Design review of the part built by this model. Coordinates are the model's own, in mm. A direction names the side the tool comes from. Round coordinates to 2 decimals unless told otherwise and drop trailing zeros. Loops run counter-clockwise (first coordinate to the right, second up) from the corner with the lowest first, then second, coordinate; pieces in that order, holes last. Notation, with made-up numbers: M 63.25,78.25 L 82.25,78.25 A31 ccw 82.25,115.25 Z; hole C -25.5,65.25 d5. An arc over 180 degrees is marked long. One line per item, written item: value. Start each with the question number.
Item 1: For faces 1 (the flat face through (68, -13.545, 8)), 2 (the flat face through (60.993, 27.798, 7.88)), 3 (the flat face through (50.546, 30, 6)), 4 (the cylindrical face through (21.97, -7.67, 1.93)), 5 (the cylindrical face through (48.735, -20.96, 1.878)), list the 3-axis set-ups (+Z, -Z, +X, -X, +Y, -Y) from which the entire face can be reached by the end or side of a thin tool; tool diameter is ignored.
Item 2: Clearance check with flat-ended pins moving along their axes: pin 1 (1.2 mm diameter, centred on x = -16.002, y = 19.05, fed in from +Z); pin 2 (3 mm diameter, centred on x = 49.5, z = 2, fed in from -Y); pin 3 (4 mm diameter, centred on x = 52, z = 1, fed in from +Y); pin 4 (8 mm diameter, centred on x = 15.24, y = -11.43, fed in from +Z). State where each tip first meets the part, or that it passes through.
Item 3: We need section B-B (z = 10.25). State how many separate pieces and enclosed holes the cut face has, then the cut area to 3 significant figures.
Item 4: We need section C-C (x = 42.5). Write out the cut boundary in (y, z) (3 decimals).
Item 5: For line 1 along Y through (x, z) = (0, 3); line 2 along Y through (x, z) = (-11, 1.75); line 3 along Y through (x, z) = (51, 7.5), list the stretches that pass through material, from the lowest coordinate up.
Item 6: We need section D-D (x = 15.24). Write out the cut boundary in (y, z) (3 decimals), then the cut area to 3 significant figures.
Item 7: We need section A-A (x = -41). Write out the cut boundary in (y, z) (3 decimals).
Item 8: Mouldability with a two-part tool opening along Y and no side actions: class faces 6 (the cylindrical face through (64.222, -32.664, 6.388)), 7 (the flat face through (1, 1, 0)), 8 (the cylindrical face through (6.5, -20.9, 1.9)) as released by +Y, released by -Y, zero draft, split by the parting line, or undercut.
from build123d import *

# Parameters (mm, degrees)
BOSS_EXTRUDE1_DEPTH     = 3.81
BOSS_EXTRUDE2_DEPTH     = 8.255
SKETCH3_W               = 64.77
SKETCH3_H               = 7.1
CUT_EXTRUDE1_DEPTH      = 0.635
CUT_EXTRUDE4_DEPTH      = 4.81
CUT_EXTRUDE5_DEPTH      = 4.81
SKETCH12_R              = 2.4257
CUT_EXTRUDE6_DEPTH      = 4.81
SKETCH4_R               = 1.143
CUT_EXTRUDE2_DEPTH      = 11.43
SKETCH17_R              = 2.413
CUT_EXTRUDE9_DEPTH      = 4.81
BOSS_EXTRUDE5_DEPTH     = 8.255
SKETCH20_W              = 69.85
SKETCH20_H              = 3.175
BOSS_EXTRUDE6_DEPTH     = 2.54
SKETCH21_R              = 1.02235
CUT_EXTRUDE10_DEPTH     = 13.065
SKETCH24_R              = 1.6383
CUT_EXTRUDE11_DEPTH     = 8.128
CIRPATTERN1_COUNT       = 2
CIRPATTERN1_ANGLE       = 15
MIRROR2_COPY_1_SKETCH_R = 1.6383
MIRROR2_COPY_1_DEPTH    = 8.128


with BuildPart() as part:
    # Sketch1 → Boss-Extrude1 (new body)
    with BuildSketch(Plane.XY):
        with BuildLine():
            Line((10.977415053, 19.05), (44.196, 19.05))
            ThreePointArc((44.196, 19.05), (48.686128061, 20.909871939), (50.546, 25.4))
            Line((50.546, 25.4), (50.546, 44.45))
            Line((50.546, 44.45), (61.579155694, 44.45))
            ThreePointArc((61.579155694, 44.45), (75.946, 0), (61.579155694, -44.45))
            Line((61.579155694, -44.45), (50.546, -44.45))
            Line((50.546, -44.45), (50.546, -25.4))
            ThreePointArc((50.546, -25.4), (48.686128061, -20.909871939), (44.196, -19.05))
            Line((44.196, -19.05), (10.977415053, -19.05))
            ThreePointArc((10.977415053, -19.05), (6.487286992, -20.909871939), (4.627415053, -25.4))
            Line((4.627415053, -25.4), (-71.572584947, -25.4))
            ThreePointArc((-71.572584947, -25.4), (-75.946, 0), (-71.572584947, 25.4))
            Line((-71.572584947, 25.4), (4.627415053, 25.4))
            ThreePointArc((4.627415053, 25.4), (6.487286992, 20.909871939), (10.977415053, 19.05))
        make_face()
    extrude(amount=BOSS_EXTRUDE1_DEPTH)

    # Sketch2 → Boss-Extrude2 (add)
    with BuildSketch(Plane.XY.offset(3.81)):
        with BuildLine():
            Line((61.865268471, 17.78), (60.095110466, 38.1))
            ThreePointArc((60.095110466, 38.1), (59.464196764, 40.158289632), (58.047089349, 41.778911391))
            Line((58.047089349, 41.778911391), (57.900800643, 44.704))
            Line((57.900800643, 44.704), (61.395010384, 44.704))
            ThreePointArc((61.395010384, 44.704), (69.822038137, 29.877715884), (74.728381149, 13.544887112))
            Line((74.728381149, 13.544887112), (60.759450402, 13.544887112))
            Line((60.759450402, 13.544887112), (60.759450402, 15.094127876))
            ThreePointArc((60.759450402, 15.094127876), (61.639191639, 16.302501703), (61.865268471, 17.78))
        make_face()
        with BuildLine():
            Line((58.651639318, 17.500047669), (56.881481313, 37.820047669))
            Line((56.881481313, 37.820047669), (50.546, 37.820047669))
            Line((50.546, 37.820047669), (50.546, 16.566735288))
            Line((50.546, 16.566735288), (57.366094516, 16.566735288))
            ThreePointArc((57.366094516, 16.566735288), (58.160401987, 16.824667019), (58.651639318, 17.500047669))
        make_face()
        with BuildLine():
            Line((60.759450402, -13.544887112), (74.728381149, -13.544887112))
            ThreePointArc((74.728381149, -13.544887112), (69.822038137, -29.877715884), (61.395010384, -44.704))
            Line((61.395010384, -44.704), (57.900800643, -44.704))
            Line((57.900800643, -44.704), (58.047089349, -41.778911391))
            ThreePointArc((58.047089349, -41.778911391), (59.464196764, -40.158289632), (60.095110466, -38.1))
            Line((60.095110466, -38.1), (61.865268471, -17.78))
            ThreePointArc((61.865268471, -17.78), (61.639191639, -16.302501703), (60.759450402, -15.094127876))
            Line((60.759450402, -15.094127876), (60.759450402, -13.544887112))
        make_face()
        with BuildLine():
            Line((50.546, -16.566735288), (57.366094516, -16.566735288))
            ThreePointArc((57.366094516, -16.566735288), (58.160401987, -16.824667019), (58.651639318, -17.500047669))
            Line((58.651639318, -17.500047669), (56.881481313, -37.820047669))
            Line((56.881481313, -37.820047669), (50.546, -37.820047669))
            Line((50.546, -37.820047669), (50.546, -16.566735288))
        make_face()
    extrude(amount=BOSS_EXTRUDE2_DEPTH)

    # Sketch3 → Cut-Extrude1 (cut)
    with BuildSketch(Plane.XY.offset(3.81)):
        with Locations((44.577, 0)):
            Rectangle(SKETCH3_W, SKETCH3_H)
    extrude(amount=-CUT_EXTRUDE1_DEPTH, mode=Mode.SUBTRACT)

    # Sketch9 → Cut-Extrude4 (cut, through all)
    with BuildSketch(Plane.XY.offset(3.81)):
        with BuildLine():
            Line((69.85, 11.17), (25.4, 11.17))
            ThreePointArc((25.4, 11.17), (21.971, 7.741), (25.4, 4.312))
            Line((25.4, 4.312), (69.85, 4.312))
            ThreePointArc((69.85, 4.312), (73.279, 7.741), (69.85, 11.17))
        make_face()
        with BuildLine():
            Line((69.85, -4.312), (25.4, -4.312))
            ThreePointArc((25.4, -4.312), (21.971, -7.741), (25.4, -11.17))
            Line((25.4, -11.17), (69.85, -11.17))
            ThreePointArc((69.85, -11.17), (73.279, -7.741), (69.85, -4.312))
        make_face()
    extrude(amount=-CUT_EXTRUDE4_DEPTH, mode=Mode.SUBTRACT)

    # Sketch10 → Cut-Extrude5 (cut, through all)
    with BuildSketch(Plane.XY.offset(3.81)):
        with BuildLine():
            Line((-10.922, 11.43), (-59.182, 11.43))
            ThreePointArc((-59.182, 11.43), (-61.42706403, 10.50006403), (-62.357, 8.255))
            Line((-62.357, 8.255), (-62.357, -8.255))
            ThreePointArc((-62.357, -8.255), (-61.42706403, -10.50006403), (-59.182, -11.43))
            Line((-59.182, -11.43), (-10.922, -11.43))
            ThreePointArc((-10.922, -11.43), (-8.67693597, -10.50006403), (-7.747, -8.255))
            Line((-7.747, -8.255), (-7.747, 8.255))
            ThreePointArc((-7.747, 8.255), (-8.67693597, 10.50006403), (-10.922, 11.43))
        make_face()
    extrude(amount=-CUT_EXTRUDE5_DEPTH, mode=Mode.SUBTRACT)

    # Sketch12 → Cut-Extrude6 (cut, through all)
    with BuildSketch(Plane.XY.offset(3.81)):
        with Locations((15.24, 11.43)):
            Circle(SKETCH12_R)
        with Locations((15.24, -11.43)):
            Circle(SKETCH12_R)
    extrude(amount=-CUT_EXTRUDE6_DEPTH, mode=Mode.SUBTRACT)

    # Sketch4 → Cut-Extrude2 (cut)
    with BuildSketch(Plane.XY.offset(3.175)):
        with Locations((19.812, 0)):
            Circle(SKETCH4_R)
        with Locations((34.798, 0)):
            Circle(SKETCH4_R)
        with Locations((49.784, 0)):
            Circle(SKETCH4_R)
        with Locations((64.77, 0)):
            Circle(SKETCH4_R)
    extrude(amount=-CUT_EXTRUDE2_DEPTH, mode=Mode.SUBTRACT)

    # Sketch17 → Cut-Extrude9 (cut, through all)
    with BuildSketch(Plane.XY.offset(3.81)):
        with Locations((-0.127, 16.51)):
            Circle(SKETCH17_R)
        with Locations((-0.127, -16.51)):
            Circle(SKETCH17_R)
    extrude(amount=-CUT_EXTRUDE9_DEPTH, mode=Mode.SUBTRACT)

    # Sketch19 → Boss-Extrude5 (add)
    with BuildSketch(Plane.XY.offset(3.81)):
        with BuildLine():
            Line((-71.572584947, -25.4), (-65.222584947, -25.4))
            Line((-65.222584947, -25.4), (-65.222584947, 25.4))
            Line((-65.222584947, 25.4), (-71.572584947, 25.4))
            ThreePointArc((-71.572584947, 25.4), (-75.946, 0), (-71.572584947, -25.4))
        make_face()
    extrude(amount=BOSS_EXTRUDE5_DEPTH)

    # Sketch20 → Boss-Extrude6 (add)
    with BuildSketch(Plane.XZ.offset(25.4)):
        with Locations((-30.297584947, 5.3975)):
            Rectangle(SKETCH20_W, SKETCH20_H)
    boss_extrude6 = extrude(amount=-BOSS_EXTRUDE6_DEPTH)

    # Mirror1: Boss-Extrude6 across plane
    add(boss_extrude6.mirror(Plane.ZX))

    # Sketch21 → Cut-Extrude10 (cut, through all)
    with BuildSketch(Plane(origin=(0, 0, 0), x_dir=(-1, 0, 0), z_dir=(0, 0, -1))):
        with Locations((54.102, 19.05)):
            Circle(SKETCH21_R)
        with Locations((16.002, 19.05)):
            Circle(SKETCH21_R)
        with Locations((16.002, -19.05)):
            Circle(SKETCH21_R)
        with Locations((54.102, -19.05)):
            Circle(SKETCH21_R)
    extrude(amount=-CUT_EXTRUDE10_DEPTH, mode=Mode.SUBTRACT)

    # Sketch24 → Cut-Extrude11 (cut)
    with BuildSketch(Plane(origin=(65.771165316, 37.973, 0), x_dir=(0, 0, -1), z_dir=(0.866025404, 0.5, 0))):
        with Locations((-6.0325, -2.224428615)):
            Circle(SKETCH24_R)
    cut_extrude11 = extrude(amount=-CUT_EXTRUDE11_DEPTH, mode=Mode.SUBTRACT)

    # CirPattern1: Cut-Extrude11 ×2 about axis
    cirpattern1_axis = Axis((0, 0, 3.81), (0, 0, -1))
    for i in range(1, CIRPATTERN1_COUNT):
        add(cut_extrude11.rotate(cirpattern1_axis, i * CIRPATTERN1_ANGLE / (CIRPATTERN1_COUNT - 1)), mode=Mode.SUBTRACT)

    # Mirror2: Cut-Extrude11 across plane
    add(cut_extrude11.mirror(Plane.ZX), mode=Mode.SUBTRACT)

    # Mirror2 copy 1 sketch → Mirror2 copy 1 (cut)
    with BuildSketch(Plane(origin=(73.358202803, -19.656271199, 0), x_dir=(0, 0, -1), z_dir=(0.965925826, -0.258819045, 0))):
        with Locations((-6.0325, 2.224428615)):
            Circle(MIRROR2_COPY_1_SKETCH_R)
    extrude(amount=-MIRROR2_COPY_1_DEPTH, mode=Mode.SUBTRACT)


solid = part.part
A:
1. face 1: +Z, +X
1. face 2: +Z
1. face 3: +Z, +Y
1. face 4: +Z, -Z
1. face 5: +Z, -Z, -Y
2. pin 1: through
2. pin 2: y = -44.45
2. pin 3: y = 44.45
2. pin 4: z = 3.81
3. separate pieces: 5
3. enclosed holes: 0
3. area: 1,330 mm2
4. outline: M -19.05,0 L -11.17,0 L -11.17,3.81 L -19.05,3.81 Z; M -4.312,0 L 4.312,0 L 4.312,3.81 L 3.55,3.81 L 3.55,3.175 L -3.55,3.175 L -3.55,3.81 L -4.312,3.81 Z; M 11.17,0 L 19.05,0 L 19.05,3.81 L 11.17,3.81 Z
5. line 1: -25.4 to -18.92, -14.1 to 14.1, 18.92 to 25.4
5. line 2: -25.4 to -11.43, 11.43 to 25.4
5. line 3: -37.82 to -16.57, 16.57 to 37.82
6. outline: M -19.05,0 L -13.856,0 L -13.856,3.81 L -19.05,3.81 Z; M -9.004,0 L 9.004,0 L 9.004,3.81 L 3.55,3.81 L 3.55,3.175 L -3.55,3.175 L -3.55,3.81 L -9.004,3.81 Z; M 13.856,0 L 19.05,0 L 19.05,3.81 L 13.856,3.81 Z
6. area: 104 mm2
7. outline: M -25.4,0 L -11.43,0 L -11.43,3.81 L -22.86,3.81 L -22.86,6.985 L -25.4,6.985 Z; M 11.43,0 L 25.4,0 L 25.4,6.985 L 22.86,6.985 L 22.86,3.81 L 11.43,3.81 Z
8. face 6: undercut
8. face 7: zero draft
8. face 8: released by -Y
